Autodesk Inventor part; units mm, degrees
ref_plane "YZ Plane" through (0, 0, 0) normal (1, 0, 0) x (0, 1, 0)
ref_plane "XZ Plane" through (0, 0, 0) normal (0, 1, 0) x (-1, 0, 0)
ref_plane "XY Plane" through (0, 0, 0) normal (0, 0, 1) x (1, 0, 0)
sketch "Sketch2" plane through (0, 0, 0) normal (0, 0, 1) x (1, 0, 0)
  circle A0 centre (0, 0) radius 3.175 construction
  circle A1 centre (0, 0) radius 7.9375 construction
  line L0 (-24.9815, -53.975) -> (30.0677, -53.975)
  line L1 (-24.9815, -53.975) -> (-36.2864, -11.7845) construction
  line L2 (-36.2864, -11.7845) -> (-3.9688, 6.8741) construction
  line L3 (20.5427, -47.625) -> (-13.5349, -47.625)
  line L4 (-13.5349, -47.625) -> (-22.3476, -14.7355) construction
  line L5 (-22.3476, -14.7355) -> (-5.9414, -5.2634) construction
  line L6 (-18.5621, -41.1307) -> (-23.4926, -22.7298) construction
  line L7 (-23.4926, -22.7298) -> (-29.6262, -24.3733) construction
  line L8 (-29.6262, -24.3733) -> (-24.6957, -42.7742) construction
  line L9 (-24.6957, -42.7742) -> (-18.5621, -41.1307) construction
  line L10 (-18.5621, -41.1307) -> (-29.6262, -24.3733) construction
  line L11 (-23.4926, -22.7298) -> (-24.6957, -42.7742) construction
  circle A2 centre (-29.6262, -24.3733) radius 1.7526 construction
  circle A3 centre (-24.6957, -42.7742) radius 1.7526 construction
  circle A4 centre (-21.0273, -31.9303) radius 1.7526 construction
  line L12 (25.3052, -45.5804) -> (25.3052, -53.975)
  circle A5 centre (25.3052, -39.2375) radius 1.7526
  line L13 (0, 0) -> (-58.6646, -15.7191) construction
  line L14 (-24.0941, -32.752) -> (-30.6681, -8.2175) construction
  circle A6 centre (25.3052, -39.2375) radius 4.7625
  line L15 (30.0677, -39.2375) -> (30.0677, -53.975)
  line L16 (20.5427, -39.2375) -> (20.5427, -47.625)
  line L17 (-30.2278, -34.3955) -> (-17.9605, -31.1085) construction
  line L18 (-24.9815, -53.975) -> (-113.8815, -53.975)
  circle A7 centre (-9.9632, -48.6877) radius 1.7526
  line L19 (-9.9632, -48.6877) -> (-25.2973, -52.7964) construction
  line L20 (25.3052, -39.2375) -> (24.0725, -34.6373)
  line L21 (-31.2313, -30.6503) -> (-77.8688, -47.625) construction
  line L22 (-77.8688, -47.625) -> (-26.6829, -47.625) construction
  line L23 (-9.9632, -48.6877) -> (-10.4168, -46.9948) construction
  circle A8 centre (25.3052, -39.2375) radius 1.7526
  circle A9 centre (25.3052, -39.2375) radius 4.7625
  line L24 (17.994, -39.5531) -> (8.9547, -5.8181) construction
  line L25 (8.9547, -5.8181) -> (-22.4801, -14.241) construction
  line L26 (-22.4801, -14.241) -> (-13.4409, -47.976) construction
  line L27 (-0.2817, -44.45) -> (17.994, -39.5531) construction
  line L28 (17.994, -39.5531) -> (-22.4801, -14.241) construction
  line L29 (8.9547, -5.8181) -> (-13.4409, -47.976) construction
  line L30 (6.9477, 3.8384) -> (29.4738, -36.9345)
  line L31 (2.0544, -7.667) -> (8.9547, -5.8181) construction
  circle A10 centre (-9.9632, -48.6877) radius 4.7625
  line L32 (-0.2817, -44.45) -> (-14.3857, -44.45) construction
  line L33 (-113.8815, -53.975) -> (-32.8811, -24.4933) construction
  circle A11 centre (-54.7623, -40.9695) radius 1.7526 construction
  circle A12 centre (-54.7623, -40.9695) radius 7.9375 construction
  line L34 (-54.7623, -40.9695) -> (-56.8404, -33.2138) construction
  line L35 (-25.8322, -50.8) -> (-105.1582, -50.8) construction
  circle A13 centre (-57.15, -50.8) radius 1.7526
  circle A14 centre (-66.675, -50.8) radius 1.7526 construction
  circle A15 centre (-76.2, -50.8) radius 1.7526 construction
  circle A16 centre (-85.725, -50.8) radius 1.7526 construction
  circle A17 centre (12.7, -50.8) radius 1.7526
  line L36 (-2.2431, -26.897) -> (20.5536, -20.7887) construction
  line L37 (25.3052, -39.2375) -> (-9.9632, -48.6877) construction
  line L38 (26.5378, -43.8377) -> (-8.7306, -53.2879)
  line L39 (-48.0967, -53.975) -> (24.0725, -34.6373)
  arc A18 (26.5378, -43.8377) -> (24.0725, -34.6373) centre (25.3052, -39.2375) ccw
  arc A19 (-11.1958, -44.0874) -> (-8.7306, -53.2879) centre (-9.9632, -48.6877) ccw
  line L40 (-36.2475, -50.8) -> (-36.2475, -53.975) construction
  line L41 (-36.2475, -50.8) -> (-38.7127, -41.5996) construction
  line L42 (-38.7127, -41.5996) -> (-84.8985, -53.975)
  circle A20 centre (-37.0692, -47.7332) radius 3.175
  line L43 (-41.7795, -42.4213) -> (-39.3143, -51.6218)
  line L44 (-38.7127, -41.5996) -> (22.9264, -25.0834)
  arc A21 (22.9264, -25.0834) -> (-12.7947, -34.6548) centre (6.2519, -34.2957) ccw
  line L45 (-39.3143, -51.6218) -> (27.6718, -33.6729) construction
  circle A22 centre (-57.15, -50.8) radius 3.175
  line L46 (-60.325, -50.8) -> (-60.325, -47.3906)
  point P0 (30.0677, -39.2375)
  point P1 (-24.0941, -32.752)
  point P2 (-2.2431, -26.897)
  point P3 (-12.1309, -47.625)
  point P4 (-15.5208, -47.3441)
  point P5 (-14.3857, -44.45)
  point P6 (-9.6568, -46.9621)
  point P7 (-9.6568, -46.9621)
  point P8 (-48.0301, -36.7646)
  point P9 (-59.0876, -47.625)
  point P10 (-62.6223, -42.0757)
  point P11 (-50.4369, -47.625)
  point P12 (0.6918, 7.9073)
  point P13 (7.671, -43.9626)
  point P14 (26.5378, -43.8377)
  point P15 (-40.136, -48.5549)
  point P16 (-57.15, -53.975)
  dimension "d40" = 3.5052
  dimension "d6" = 6.35
  dimension "d7" = 15.875
  dimension "Angle_Mount" = 105
  dimension "d17" = 105
  dimension "d19" = 9.525
  dimension "d20" = 12.7
  dimension "d24" = 19.05
  dimension "d25" = 6.35
  dimension "d26" = 3.5052
  dimension "d27" = 3.5052
  dimension "d28" = 3.5052
  dimension "d29" = 6.35
  dimension "d33" = 3.5052
  dimension "d35" = 31.75
  dimension "d37" = 9.525
  dimension "d38" = 25.4
  dimension "d39" = 53.975
  dimension "d41" = 44.45
  dimension "Rail_Offset" = 36.5125
  dimension "d45" = 6.35
  dimension "d48" = 22.225
  dimension "d49" = 3.5052
  dimension "d51" = 9.525
  dimension "d52" = 32.5438
  dimension "d53" = 34.925
  dimension "d54" = 9.525
  dimension "d56" = 9.525
  dimension "d58" = 6.35
  dimension "d60" = 20
  dimension "d61" = 88.9
  dimension "d69" = 31.75
  dimension "d71" = 3.5052
  dimension "d72" = 15.875
  dimension "d74" = 3.175
  dimension "d75" = 3.5052
  dimension "d76" = 57.15
  dimension "d79" = 9.525
  dimension "d84" = 3.5052
  dimension "d85" = 69.85
  dimension "d106" = 3.175
  dimension "d107" = 9.525
  dimension "d109" = 6.35
  dimension "d113" = 19.05
  dimension "d122" = 9.525
extrude "Extrusion2" add sketch "Sketch2" along normal blind 9.525 contours L18 L39 A10 L38 L3 L16 A6 L15 L0 | L18 A22 L46 L42 L43 L39 | A22 | A6 | L38 L16 A6 | A10 | L39 A6 L16 L38 L3 A10 | L16 L3 L38 | A10 L3 L38 | A7 L3 | L3 A7 | A5
extrude "Extrusion3" add sketch "Sketch2" along normal blind 3.175 contours L43 A20 L39 | A20 L43 L42 L44 L30 A6 L39 | A20 | L38 L16 A6 | A10 | L39 A6 L16 L38 L3 A10 | L44 A21 | A10 L3 L38 | A7 L3 | L3 A7
fillet "Fillet6" radius 6.35 3 edges at (22.9264, -25.0834, 1.5875) (-12.7947, -34.6548, 1.5875) (29.4738, -36.9345, 1.5875)
fillet "Fillet7" radius 3.175 2 edges at (-39.3143, -51.6218, 6.35) (-60.325, -47.3906, 4.7625)
properties part number "Uprights" material "UHMW, White"
Build history of the part. All positions in model axes, mm. A direction names the side the tool comes from. Coordinates: 2 decimals unless noted, no trailing zeros. Order: outer loops, then holes, each group sorted by start corner. A loop starts at its lowest first (then second) coordinate and runs counter-clockwise, first axis right, second up. Notation, with made-up numbers: (63, 79) -> (86, 79) arc R5 ccw to (86, 83) -> close; hole circle Ø7 at (46, -28). An arc over 180 degrees is marked (long way). One line per item, written item: value.
(1) Drop a flat-ended pin along its axis: pin 1 Ø1 at (x, z) = (21, 5.5) entering from +Y. Give the stop position or say it passes through.
Checked values:
pin 1: y = -35.33
(2) Slice it at D-D, the plane x = -8.5. List the corners of the cut face in (y, z) (3 decimals), plus the area to 3 significant figures.
Checked values:
outline: (-53.975, 0) -> (-22.242, 0) -> (-22.242, 3.175) -> (-43.365, 3.175) -> (-43.365, 9.525) -> (-53.975, 9.525) -> close
area: 168 mm2
(3) Tool access for faces 4 (the flat face through (-6.51, -42.83, 6.31)), 5 (the flat face through (-13, -53.975, 5)): list every direction of +Z, -Z, +X, -X, +Y, -Y with a clear straight run to the whole face (end or side of a thin tool).
Checked values:
face 4: +Z, +Y
face 5: +Z, -Z, +X, -X, -Y
(4) Slice it at A-A, the plane z = 4.75. Count the separate pieces of the cut face and the enclosed holes in it, plus the area to 3 significant figures.
Checked values:
separate pieces: 1
enclosed holes: 2
area: 964 mm2
(5) Mould opens along X. For faces 1 (the flat face through (-6, -39, 0)), 2 (the cylindrical face through (-59.37, -53.07, 4.7)), 3 (the flat face through (-40.97, -45.45, 6.31)) say: pulls with the +X half, pulls with the -X half, needs draft (parallel to the pull), parting line crosses it, or undercut.
Checked values:
face 1: needs draft
face 2: pulls with the -X half
face 3: undercut
(6) Slice it at B-B, the plane x = 12.7. List the corners of the cut face in (y, z) (3 decimals), plus the area to 3 significant figures.
Checked values:
outline: (-53.975, 0) -> (-52.553, 0) -> (-52.553, 9.525) -> (-53.975, 9.525) -> close; (-49.047, 0) -> (-16.37, 0) -> (-16.37, 3.175) -> (-37.685, 3.175) -> (-37.685, 9.525) -> (-49.047, 9.525) -> close
area: 189 mm2
(7) Probe line 1 (X direction, y = -51, z = 9); line 2 (Z direction, x = -13, y = -40) (3 decimals); line 3 (Y direction, x = -57.15, z = 2.75) (3 decimals). List the from-to ranges inside material, lowest first. Write a range as [from, to].
Checked values:
line 1: [-60.32, -58.89], [-55.41, 10.96], [14.44, 30.07]
line 2: [0, 3.175]
line 3: [-53.975, -52.553], [-49.047, -46.54]
(8) Slice it at C-C, the plane y = -44. List the corners of the cut face in (x, z) (1 decimal), plus the area to 3 significant figures.
Checked values:
outline: (-47.7, 0) -> (30.1, 0) -> (30.1, 9.5) -> (-10.9, 9.5) -> (-10.9, 3.2) -> (-41.4, 3.2) -> (-41.4, 9.5) -> (-47.7, 9.5) -> close
area: 547 mm2
